Source: CAD feature listing. Evaluate the final solid. Frame: model axes, mm. Round coordinates to 2 decimals unless told otherwise and drop trailing zeros. Write each loop counter-clockwise with the first axis right and the second up, starting at its lowest first coordinate (ties: lowest second). Pieces come first, ordered by that corner, then holes. Notation, with made-up numbers: M 27,7 L 76,7 A11 ccw 76,26 Z; hole C 89,35.5 d2. An arc over 180 degrees is marked long. Answer in a Markdown table with one row per item. Add a question column.
Item 1: Material intervals for probe 1 along X at (y, z) = (39.75, 2.95) (3 decimals); probe 2 along Y at (x, z) = (126.5, 1); probe 3 along Y at (x, z) = (147.5, 3.35) (3 decimals), sorted ascending.
Item 2: Contact query for flat-ended pins moving along their axis: pin 1 (3.5 mm diameter, centred on x = 45, y = 45, fed in from -Z); pin 2 (1.5 mm diameter, centred on y = 45, z = 3.5, fed in from -X); pin 3 (1.5 mm diameter, centred on x = 15, y = 6, fed in from +Z); pin 4 (0.8 mm diameter, centred on y = 12.5, z = 3.5, fed in from -X). Output: stop coordinate, or through.
Item 3: Cut plane B-B on y = 24. Return loops of the section in (x, z).
Item 4: Cut plane A-A on x = 95. Return loops of the section in (y, z).
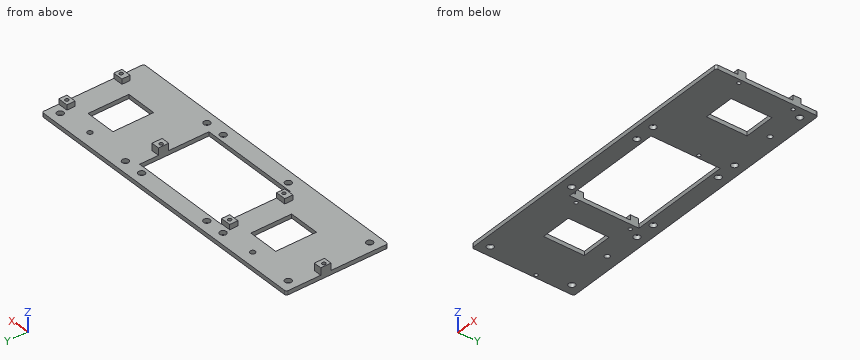
from build123d import *

# Parameters (mm, degrees)
SKETCH_W        = 150
SKETCH_H        = 50
SKETCH_R        = 1.6
SKETCH_R_2      = 1.23
SKETCH_W_2      = 50
SKETCH_H_2      = 34
SKETCH_W_3      = 15.25
SKETCH_H_3      = 20
PAD_DEPTH       = 2
SKETCH001_W     = 5
SKETCH001_H     = 4
SKETCH001_W_2   = 4
SKETCH001_H_2   = 5
PAD001_DEPTH    = 3.5
SKETCH002_R     = 0.875
POCKET_DEPTH    = 5.5
SKETCH003_W     = 5
SKETCH003_H     = 4
POCKET001_DEPTH = 1
FILLET_R        = 1


with BuildPart() as part:
    # Sketch → Pad (new body)
    with BuildSketch(Plane.XY):
        with Locations((75, 25)):
            Rectangle(SKETCH_W, SKETCH_H)
        with Locations((5, 45)):
            Circle(SKETCH_R, mode=Mode.SUBTRACT)
        with Locations((5, 5)):
            Circle(SKETCH_R, mode=Mode.SUBTRACT)
        with Locations((45, 45)):
            Circle(SKETCH_R, mode=Mode.SUBTRACT)
        with Locations((55, 45)):
            Circle(SKETCH_R, mode=Mode.SUBTRACT)
        with Locations((55, 5)):
            Circle(SKETCH_R, mode=Mode.SUBTRACT)
        with Locations((95, 45)):
            Circle(SKETCH_R, mode=Mode.SUBTRACT)
        with Locations((105, 45)):
            Circle(SKETCH_R, mode=Mode.SUBTRACT)
        with Locations((95, 5)):
            Circle(SKETCH_R, mode=Mode.SUBTRACT)
        with Locations((105, 5)):
            Circle(SKETCH_R, mode=Mode.SUBTRACT)
        with Locations((145, 45)):
            Circle(SKETCH_R, mode=Mode.SUBTRACT)
        with Locations((128.1, 43.95)):
            Circle(SKETCH_R_2, mode=Mode.SUBTRACT)
        with Locations((28.1, 43.95)):
            Circle(SKETCH_R_2, mode=Mode.SUBTRACT)
        with Locations((75, 25)):
            Rectangle(SKETCH_W_2, SKETCH_H_2, mode=Mode.SUBTRACT)
        with Locations((30.625, 26.75)):
            Rectangle(SKETCH_W_3, SKETCH_H_3, mode=Mode.SUBTRACT)
        with Locations((130.625, 26.75)):
            Rectangle(SKETCH_W_3, SKETCH_H_3, mode=Mode.SUBTRACT)
    extrude(amount=PAD_DEPTH)

    # Sketch001 (on Face30 of Pad) → Pad001 (join)
    with BuildSketch(Plane.XY.offset(2)):
        with Locations((47.5, 39.75)):
            Rectangle(SKETCH001_W, SKETCH001_H)
        with Locations((47.5, 12.75)):
            Rectangle(SKETCH001_W, SKETCH001_H)
        with Locations((2, 30.5)):
            Rectangle(SKETCH001_W_2, SKETCH001_H_2)
        with Locations((147.5, 39.75)):
            Rectangle(SKETCH001_W, SKETCH001_H)
        with Locations((147.5, 12.75)):
            Rectangle(SKETCH001_W, SKETCH001_H)
        with Locations((102, 30.25)):
            Rectangle(SKETCH001_W_2, SKETCH001_H_2)
    extrude(amount=PAD001_DEPTH)

    # Sketch002 (on Face58 of Pad001) → Pocket (cut)
    with BuildSketch(Plane.XY.offset(5.5)):
        with Locations((47.5, 39.75)):
            Circle(SKETCH002_R)
        with Locations((48, 12.75)):
            Circle(SKETCH002_R)
        with Locations((101.5, 30.25)):
            Circle(SKETCH002_R)
        with Locations((1.5, 30.25)):
            Circle(SKETCH002_R)
        with Locations((147.5, 39.75)):
            Circle(SKETCH002_R)
        with Locations((148, 12.75)):
            Circle(SKETCH002_R)
    extrude(amount=-POCKET_DEPTH, mode=Mode.SUBTRACT)

    # Sketch003 (on Face62 of Pocket) → Pocket001 (cut)
    with BuildSketch(Plane.XY.offset(5.5)):
        with Locations((47.5, 39.75)):
            Rectangle(SKETCH003_W, SKETCH003_H)
        with Locations((47.5, 12.75)):
            Rectangle(SKETCH003_W, SKETCH003_H)
        with Locations((147.5, 12.75)):
            Rectangle(SKETCH003_W, SKETCH003_H)
        with Locations((147.5, 39.75)):
            Rectangle(SKETCH003_W, SKETCH003_H)
    extrude(amount=-POCKET001_DEPTH, mode=Mode.SUBTRACT)

    # Fillet
    fillet_edges = [part.edges().sort_by_distance(p)[0] for p in [
        (0, 0, 1),
        (0, 50, 1),
        (150, 0, 1),
        (150, 50, 1),
    ]]
    fillet(fillet_edges, radius=FILLET_R)


solid = part.part
Results below:
| question | item | result |
|---|---|---|
| 1 | probe 1 | 45 to 46.625, 48.375 to 50, 145 to 146.625, 148.375 to 150 |
| 1 | probe 2 | 0 to 16.75, 36.75 to 50 |
| 1 | probe 3 | 10.75 to 12.032, 13.468 to 14.75, 37.75 to 38.875, 40.625 to 41.75 |
| 2 | pin 1 | z = 0 |
| 2 | pin 2 | through |
| 2 | pin 3 | z = 2 |
| 2 | pin 4 | x = 45 |
| 3 | outline | M 0,0 L 23,0 L 23,2 L 0,2 Z; M 38.25,0 L 50,0 L 50,2 L 38.25,2 Z; M 100,0 L 123,0 L 123,2 L 100,2 Z; M 138.25,0 L 150,0 L 150,2 L 138.25,2 Z |
| 4 | outline | M 0,0 L 3.4,0 L 3.4,2 L 0,2 Z; M 6.6,0 L 8,0 L 8,2 L 6.6,2 Z; M 42,0 L 43.4,0 L 43.4,2 L 42,2 Z; M 46.6,0 L 50,0 L 50,2 L 46.6,2 Z |
